Build history of the part. All positions in model axes, mm. Face numbers are marked on the shaded views. A direction names the side the tool comes from. Give positions to 0.01 mm unless a question says otherwise; leave off trailing zeros. Order: outer loops, then holes, each group sorted by start corner. A loop starts at its lowest first (then second) coordinate and runs counter-clockwise, first axis right, second up. Notation, with made-up numbers: (70, 20) - (84, 20) arc R34 ccw to (84, 59) - close; hole circle Ø7 at (53.5, 64.25). An arc over 180 degrees is marked (long way). Use a Markdown table: item, result. Add a question column.
(1) Slice it at A-A (x = 0). Write the cut outline in (y, z).
(2) Which spindle directions (+Z, -Z, +X, -X, +Y, -Y) get a long thin tool onto all of the face, cutting with end or side? Do the marked faces 1 and 2. Say none if no direction does.
(3) Flat gauge pins, fed straight in: pin 1 (4 mm diameter, centred on x = 3.5, z = 32.5, fed in from +Y); pin 2 (5 mm diameter, centred on y = 3.5, z = 31, fed in from +X); pin 3 (4 mm diameter, centred on x = -4, z = 30, fed in from +Y). Where does each tip first touch, or does it go through?
(4) Slice it at C-C (z = 34.25). Write the cut outline in (x, y).
(5) Wall check: line 1 (Z direction, x = -3, y = 3); line 2 (Y direction, x = -3.5, z = 30.5); line 3 (X direction, y = -3.25, z = 33.5). Give the ranges that are in metal, low to high.
(6) Slice it at D-D (z = 31). Write the cut outline in (x, y).
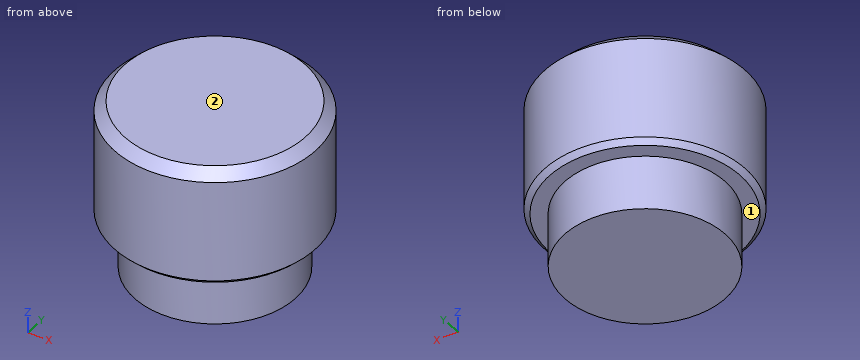
from build123d import *

# Parameters (mm, degrees)
SKETCH004_R     = 4
PAD003_DEPTH    = 2.7
SKETCH005_R     = 5
PAD004_DEPTH    = 5.8
CHAMFER_SIZE    = 0.5
CHAMFER002_SIZE = 0.25


with BuildPart() as part:
    # Sketch004 (on Face1 of CopySubtractivePipe) → Pad003 (new body)
    with BuildSketch(Plane(origin=(0, 0, 26), x_dir=(0, 1, 0), z_dir=(0, 0, 1))):
        Circle(SKETCH004_R)
    extrude(amount=PAD003_DEPTH)

    # Sketch005 (on Face3 of Pad003) → Pad004 (join)
    with BuildSketch(Plane(origin=(0, 0, 28.7), x_dir=(0, 1, 0), z_dir=(0, 0, 1))):
        Circle(SKETCH005_R)
    extrude(amount=PAD004_DEPTH)

    # Chamfer
    chamfer_edges = [part.edges().sort_by_distance(p)[0] for p in [
        (0, -5, 34.5),
    ]]
    chamfer(chamfer_edges, length=CHAMFER_SIZE)

    # Chamfer002
    chamfer002_edges = [part.edges().sort_by_distance(p)[0] for p in [
        (0, -5, 28.7),
    ]]
    chamfer(chamfer002_edges, length=CHAMFER002_SIZE)


solid = part.part
Solution:
| question | item | result |
|---|---|---|
| 1 | outline | (-5, 28.95) - (-4.75, 28.7) - (-4, 28.7) - (-4, 26) - (4, 26) - (4, 28.7) - (4.75, 28.7) - (5, 28.95) - (5, 34) - (4.5, 34.5) - (-4.5, 34.5) - (-5, 34) - close |
| 2 | face 1 | -Z |
| 2 | face 2 | +Z, +X, -X, +Y, -Y |
| 3 | pin 1 | y = 4.77 |
| 3 | pin 2 | x = 4.9 |
| 3 | pin 3 | y = 4.58 |
| 4 | outline | circle Ø9.5 at (0, 0) |
| 5 | line 1 | 28.7 to 34.5 |
| 5 | line 2 | -3.57 to 3.57 |
| 5 | line 3 | -3.8 to 3.8 |
| 6 | outline | circle Ø10 at (0, 0) |
